Geometry: final body of the model. Coordinates: model frame, mm. A direction names the side the tool comes from. Coordinates: 2 decimals unless noted, no trailing zeros. Loops run counter-clockwise (first coordinate to the right, second up) from the corner with the lowest first, then second, coordinate; pieces in that order, holes last. Notation, with made-up numbers: (44, 83) - (93, 83) arc R20 cw to (93, 108) - close; hole circle Ø11 at (53, 17). An arc over 180 degrees is marked (long way). Answer in a Markdown table with one row per item.
from build123d import *

# Parameters (mm, degrees)
SKETCH_1_W           = 55
SKETCH_1_H           = 47
EXTRUDE_1_DEPTH      = 3
SKETCH_2_W           = 4
SKETCH_2_H           = 40
EXTRUDE_2_DEPTH      = 48
SKETCH_3_R           = 1.8
CUT_EXTRUDE_1_DEPTH  = 12
SKETCH_4_R           = 1.8
SKETCH_4_R_2         = 12.5
CUT_EXTRUDE_2_DEPTH  = 12
SKETCH_5_W           = 15
SKETCH_5_H           = 30
CUT_EXTRUDE_3_DEPTH  = 12
FILLET_1_R           = 10
FILLET_2_R           = 4
CHAMFER_1_SIZE       = 5
EXTRUDE_START        = -12
EXTRUDE_3_DEPTH      = 16
EXTRUDE_4_DEPTH      = 26
EXTRUDE_4_DEPTH_BACK = 15
SKETCH_7_W           = 3.8
SKETCH_7_H           = 15
FILLET_3_R           = 1.5
SKETCH_8_W           = 4
SKETCH_8_H           = 12
EXTRUDE_5_DEPTH      = 3.8
SKETCH_9_W           = 20
SKETCH_9_H           = 2
EXTRUDE_6_DEPTH      = 23
EXTRUDE_7_DEPTH      = 2.7
SKETCH_11_R          = 1.5
CUT_EXTRUDE_4_DEPTH  = 23
FILLET_4_R           = 3
EXTRUDE_START_2      = -4
SKETCH_12_W          = 2
SKETCH_12_H          = 3
EXTRUDE_8_DEPTH      = 4
FILLET_5_R           = 1


with BuildPart() as part:
    # Эскиз1 → Бобышка-Вытянуть1 (new body)
    with BuildSketch(Plane(origin=(0, 0, 0), x_dir=(1, 0, 0), z_dir=(0, 1, 0))):
        with Locations((27.5, 23.5)):
            Rectangle(SKETCH_1_W, SKETCH_1_H)
    extrude(amount=EXTRUDE_1_DEPTH)

    # Эскиз2 → Бобышка-Вытянуть2 (add)
    with BuildSketch(Plane(origin=(-5.991084473, 3, 0), x_dir=(1, 0, 0), z_dir=(0, 1, 0))):
        with Locations((29.991084473, 22.3)):
            Rectangle(SKETCH_2_W, SKETCH_2_H)
    extrude(amount=EXTRUDE_2_DEPTH)

    # Эскиз3 → Вырез-Вытянуть1 (cut)
    with BuildSketch(Plane(origin=(0, 3, 0), x_dir=(1, 0, 0), z_dir=(0, 1, 0))):
        with Locations(Location((7, 12.45, 0), (0, 0, 270))):
            Circle(SKETCH_3_R)
        with Locations(Location((48, 12.45, 0), (0, 0, 270))):
            Circle(SKETCH_3_R)
    extrude(amount=-CUT_EXTRUDE_1_DEPTH, mode=Mode.SUBTRACT)

    # Эскиз4 → Вырез-Вытянуть2 (cut)
    with BuildSketch(Plane(origin=(26, 0, 0), x_dir=(0, 0, -1), z_dir=(1, 0, 0))):
        with Locations((6.8, 46.5)):
            Circle(SKETCH_4_R)
        with Locations((37.8, 46.5)):
            Circle(SKETCH_4_R)
        with Locations((6.8, 15.5)):
            Circle(SKETCH_4_R)
        with Locations((37.8, 15.5)):
            Circle(SKETCH_4_R)
        with Locations((22.3, 31)):
            Circle(SKETCH_4_R_2)
    extrude(amount=-CUT_EXTRUDE_2_DEPTH, mode=Mode.SUBTRACT)

    # Эскиз5 → Вырез-Вытянуть3 (cut)
    with BuildSketch(Plane(origin=(0, 3, 0), x_dir=(1, 0, 0), z_dir=(0, 1, 0))):
        with Locations((33.5, 23)):
            Rectangle(SKETCH_5_W, SKETCH_5_H)
    extrude(amount=-CUT_EXTRUDE_3_DEPTH, mode=Mode.SUBTRACT)

    # Скругление1
    fillet_1_edges = [part.edges().sort_by_distance(p)[0] for p in [
        (0, 1.5, -47),
        (55, 1.5, -47),
        (55, 1.5, 0),
    ]]
    fillet(fillet_1_edges, radius=FILLET_1_R)

    # Скругление2
    fillet_2_edges = [part.edges().sort_by_distance(p)[0] for p in [
        (24, 51, -2.3),
        (24, 51, -42.3),
    ]]
    fillet(fillet_2_edges, radius=FILLET_2_R)

    # Фаска1
    chamfer_1_edges = [part.edges().sort_by_distance(p)[0] for p in [
        (26, 3, -5.15),
        (26, 3, -40.15),
    ]]
    chamfer(chamfer_1_edges, length=CHAMFER_1_SIZE)

    # Эскиз6 → Бобышка-Вытянуть3 (add)
    with BuildSketch(Plane(origin=(0, 0, -42.3), x_dir=(-1, 0, 0), z_dir=(0, 0, -1)).offset(EXTRUDE_START)):
        Polygon((-22, 3), (-22, 7), (-17, 3), align=None)
    extrude(amount=-EXTRUDE_3_DEPTH)

    # Эскиз7 → Бобышка-Вытянуть4 (add, two sides: drawn at the far end of the back side and taken through both)
    with BuildSketch(Plane(origin=(0, 0, 0), x_dir=(0, 0, -1), z_dir=(1, 0, 0)).offset(-EXTRUDE_4_DEPTH_BACK)):
        with Locations((-1.9, 7.5)):
            Rectangle(SKETCH_7_W, SKETCH_7_H)
    extrude(amount=EXTRUDE_4_DEPTH + EXTRUDE_4_DEPTH_BACK)

    # Скругление3
    fillet_3_edges = [part.edges().sort_by_distance(p)[0] for p in [
        (5.5, 15, 0),
        (5.5, 0, 3.8),
        (5.5, 15, 3.8),
        (-7.5, 0, 0),
        (13, 3, 0),
    ]]
    fillet(fillet_3_edges, radius=FILLET_3_R)

    # Эскиз8 → Бобышка-Вытянуть5 (add)
    with BuildSketch(Plane.XY.offset(-2.3)):
        with Locations((24, 9)):
            Rectangle(SKETCH_8_W, SKETCH_8_H)
    extrude(amount=EXTRUDE_5_DEPTH)

    # Эскиз9 → Бобышка-Вытянуть6 (add)
    with BuildSketch(Plane(origin=(0, 3, 0), x_dir=(1, 0, 0), z_dir=(0, 1, 0))):
        with Locations((24, 46)):
            Rectangle(SKETCH_9_W, SKETCH_9_H)
    extrude(amount=EXTRUDE_6_DEPTH)

    # Эскиз10 → Бобышка-Вытянуть7 (add)
    with BuildSketch(Plane(origin=(0, 0, -42.3), x_dir=(-1, 0, 0), z_dir=(0, 0, -1))):
        Polygon((-22, 26), (-26, 26), (-26, 8), (-31, 3), (-22, 3), align=None)
    extrude(amount=EXTRUDE_7_DEPTH)

    # Эскиз11 → Вырез-Вытянуть4 (cut)
    with BuildSketch(Plane(origin=(0, 0, -47), x_dir=(-1, 0, 0), z_dir=(0, 0, -1))):
        with Locations((-29, 15)):
            Circle(SKETCH_11_R)
        with Locations((-19, 15)):
            Circle(SKETCH_11_R)
    extrude(amount=-CUT_EXTRUDE_4_DEPTH, mode=Mode.SUBTRACT)

    # Скругление4
    fillet_4_edges = [part.edges().sort_by_distance(p)[0] for p in [
        (14, 26, -46),
        (34, 26, -46),
    ]]
    fillet(fillet_4_edges, radius=FILLET_4_R)

    # Эскиз12 → Бобышка-Вытянуть8 (add)
    with BuildSketch(Plane.ZY.offset(-22).offset(EXTRUDE_START_2)):
        Polygon((-32.382601146, 56), (-32.382601146, 54), (-30.382601146, 54), (-26.382601146, 54), (-24.382601146, 54), (-24.382601146, 56), align=None)
        with Locations((-31.382601146, 52.5)):
            Rectangle(SKETCH_12_W, SKETCH_12_H)
        with Locations((-25.382601146, 52.5)):
            Rectangle(SKETCH_12_W, SKETCH_12_H)
    extrude(amount=EXTRUDE_8_DEPTH)

    # Скругление5
    fillet_5_edges = [part.edges().sort_by_distance(p)[0] for p in [
        (24, 54, -26.382601146),
        (24, 54, -30.382601146),
        (24, 56, -32.382601146),
        (24, 56, -24.382601146),
    ]]
    fillet(fillet_5_edges, radius=FILLET_5_R)


solid = part.part
(1) Cut plane C-C on x = 29. Output: boundary loops of the cut face in (y, z).
Verdict:
| item | result |
|---|---|
| outline | (0, -47) - (13.5, -47) - (13.5, -45) - (5, -45) - (5, -38) - (0, -38) - close; (0, -8) - (5, -8) - (5, -2.3) - (3, -2.3) - (3, 0) - (0, 0) - close; (16.5, -47) - (26, -47) - (26, -45) - (16.5, -45) - close |
(2) Ray query, probe 1 along Y at (x, z) = (24.4, -37.8); probe 2 along Z at (x, y) = (33, 2); probe 3 along Y at (x, z) = (24, -22). Return the intervals inside material, ascending.
Verdict:
| item | result |
|---|---|
| probe 1 | y = 0 to 13.7, 17.3 to 44.7, 48.3 to 51 |
| probe 2 | z = -47 to -38, -8 to 0 |
| probe 3 | y = 0 to 18.5, 43.5 to 51 |
(3) First-contact query: pin 1 Ø5 at (y, z) = (23, -40) entering from -X; pin 2 Ø9 at (x, y) = (36, 3.5) entering from +Z; pin 3 Ø1.4 at (x, z) = (11, -1) entering from +Y; pin 4 Ø3 at (y, z) = (15.5, -37.8) entering from +X. Flat tips, straight axial feed; report the tip coordinate or a pass-through.
Verdict:
| item | result |
|---|---|
| pin 1 | stops at x = 22 |
| pin 2 | stops at z = 0 |
| pin 3 | stops at y = 3.6 |
| pin 4 | passes through |
(4) Cut plane B-B on y = 31. Output: boundary loops of the cut face in (x, z), then the cut area to 3 significant figures.
Verdict:
| item | result |
|---|---|
| outline | (22, -42.3) - (26, -42.3) - (26, -34.8) - (22, -34.8) - close; (22, -9.8) - (26, -9.8) - (26, -2.3) - (22, -2.3) - close |
| area | 60.0 mm² |
(5) Cut plane A-A on z = -22.3. Output: boundary loops of the cut face in (x, y).
Verdict:
| item | result |
|---|---|
| outline | (0, 0) - (26, 0) - (26, 18.5) - (22, 18.5) - (22, 7) - (17, 3) - (0, 3) - close; (22, 43.5) - (26, 43.5) - (26, 51) - (22, 51) - close; (41, 0) - (55, 0) - (55, 3) - (41, 3) - close |
(6) Access query for faces 5 (the face through (24, 51, -35)), 6 (the face through (24, 52, -26.383)), 7 (the face through (24, 51, -15)). Directions: +Z, -Z, +X, -X, +Y, -Y. A direction counts if a zero-diameter tool reaches every point of the face in a straight line with its end or side. Return the directions, or none.
Verdict:
| item | result |
|---|---|
| face 5 | -Z, +X, -X, +Y |
| face 6 | +X, -X |
| face 7 | +Z, +X, -X, +Y |
(7) Pull-direction query (X, two-part tool) for faces 1 (the face through (3, 7, 0)), 2 (the face through (51.99, 1.52, -44.15)), 3 (the face through (20.5, 15.07, -46.01)), 4 (the face through (19.5, 5, -22.4)); classes: pulls with the +X half, pulls with the -X half, needs draft (parallel to the pull), parting line crosses it, or undercut.
Verdict:
| item | result |
|---|---|
| face 1 | needs draft |
| face 2 | pulls with the +X half |
| face 3 | undercut |
| face 4 | pulls with the -X half |
(8) Cut plane D-D on x = 48. Output: boundary loops of the cut face in (y, z), then the cut area to 3 significant figures.
Verdict:
| item | result |
|---|---|
| outline | (0, -46.54) - (3, -46.54) - (3, -14.25) - (0, -14.25) - close; (0, -10.65) - (3, -10.65) - (3, -0.46) - (0, -0.46) - close |
| area | 127 mm² |
